```python
from build123d import *

# Parameters (mm, degrees)
SKETCH1_R           = 48.9
SKETCH1_R_2         = 45.9
BOSS_EXTRUDE1_DEPTH = 2
SKETCH2_R           = 1.5
BOSS_EXTRUDE2_DEPTH = 2
SKETCH3_R           = 2.38125
BOSS_EXTRUDE3_DEPTH = 2
FILLET1_R           = 3


with BuildPart() as part:
    # Sketch1 → Boss-Extrude1 (new body)
    with BuildSketch(Plane(origin=(0, 0, 0), x_dir=(1, 0, 0), z_dir=(0, 1, 0))):
        with Locations(Location((0, 0, 0), (0, 0, 270))):
            Circle(SKETCH1_R)
        with Locations(Location((0, 0, 0), (0, 0, 270))):
            Circle(SKETCH1_R_2, mode=Mode.SUBTRACT)
    extrude(amount=BOSS_EXTRUDE1_DEPTH)

    # Sketch2 → Boss-Extrude2 (add)
    # profile 1 of 4: a face of its own
    with BuildSketch(Plane.XZ):
        with BuildLine():
            Line((-3.5, 45.766363194), (-3.5, 42.4))
            ThreePointArc((-3.5, 42.4), (0, 38.9), (3.5, 42.4))
            Line((3.5, 42.4), (3.5, 45.766363194))
            ThreePointArc((3.5, 45.766363194), (0, 45.9), (-3.5, 45.766363194))
        make_face()
        with Locations(Location((0, 42.4, 0), (0, 0, 270))):
            Circle(SKETCH2_R, mode=Mode.SUBTRACT)
    # profile 2 of 4: a face of its own
    with BuildSketch(Plane.XZ):
        with BuildLine():
            ThreePointArc((45.9, 0), (45.866578631, 1.751275164), (45.766363194, 3.5))
            Line((45.766363194, 3.5), (42.4, 3.5))
            ThreePointArc((42.4, 3.5), (38.9, 0), (42.4, -3.5))
            Line((42.4, -3.5), (45.766363194, -3.5))
            ThreePointArc((45.766363194, -3.5), (45.866578631, -1.751275164), (45.9, 0))
        make_face()
        with Locations(Location((42.4, 0, 0), (0, 0, 270))):
            Circle(SKETCH2_R, mode=Mode.SUBTRACT)
    # profile 3 of 4: a face of its own
    with BuildSketch(Plane.XZ):
        with BuildLine():
            Line((-3.5, -42.4), (-3.5, -45.766363194))
            ThreePointArc((-3.5, -45.766363194), (0, -45.9), (3.5, -45.766363194))
            Line((3.5, -45.766363194), (3.5, -42.4))
            ThreePointArc((3.5, -42.4), (0, -38.9), (-3.5, -42.4))
        make_face()
        with Locations(Location((0, -42.4, 0), (0, 0, 270))):
            Circle(SKETCH2_R, mode=Mode.SUBTRACT)
    # profile 4 of 4: a face of its own
    with BuildSketch(Plane.XZ):
        with BuildLine():
            Line((-42.4, 3.5), (-45.766363194, 3.5))
            ThreePointArc((-45.766363194, 3.5), (-45.9, 0), (-45.766363194, -3.5))
            Line((-45.766363194, -3.5), (-42.4, -3.5))
            ThreePointArc((-42.4, -3.5), (-38.9, 0), (-42.4, 3.5))
        make_face()
        with Locations(Location((-42.4, 0, 0), (0, 0, 270))):
            Circle(SKETCH2_R, mode=Mode.SUBTRACT)
    extrude(amount=-BOSS_EXTRUDE2_DEPTH)

    # Sketch3 → Boss-Extrude3 (add)
    with BuildSketch(Plane.XZ):
        with BuildLine():
            ThreePointArc((35.406018707, 29.209995537), (32.456201256, 32.456201256), (29.209995537, 35.406018707))
            Line((29.209995537, 35.406018707), (26.260178086, 32.456201256))
            ThreePointArc((26.260178086, 32.456201256), (26.260178086, 26.260178086), (32.456201256, 26.260178086))
            Line((32.456201256, 26.260178086), (35.406018707, 29.209995537))
        make_face()
        with Locations(Location((29.358189671, 29.358189671, 0), (0, 0, 270))):
            Circle(SKETCH3_R, mode=Mode.SUBTRACT)
    extrude(amount=-BOSS_EXTRUDE3_DEPTH)

    # Fillet1
    fillet1_edges = [part.edges().sort_by_distance(p)[0] for p in [
        (3.5, 1, 45.766363194),
        (-3.5, 1, 45.766363194),
        (45.766363194, 1, -3.5),
        (45.766363194, 1, 3.5),
        (-3.5, 1, -45.766363194),
        (3.5, 1, -45.766363194),
        (-45.766363194, 1, 3.5),
        (-45.766363194, 1, -3.5),
        (35.406018707, 1, 29.209995537),
        (29.209995537, 1, 35.406018707),
    ]]
    fillet(fillet1_edges, radius=FILLET1_R)


solid = part.part
```
Check sheet for the modelled part. Datum: model origin and axes. Units: mm. Give positions to 0.01 mm unless a question says otherwise; leave off trailing zeros. Order: outer loops, then holes, each group sorted by start corner. A loop starts at its lowest first (then second) coordinate and runs counter-clockwise, first axis right, second up. Notation, with made-up numbers: M 20,83.25 L 68,83.25 A18 ccw 68,104.25 Z; hole C 34.5,79.25 d6. An arc over 180 degrees is marked long. Answer in a Markdown table with one row per item. Add a question column.
Q1. Gauge pin test, flat ends, axial feed: pin 1 Ø12 at (x, z) = (16, 33.5) entering from -Y; pin 2 Ø1 at (y, z) = (1, 12) entering from -X. Record the tip position at first contact, or that the pin passes through.
Q2. Thickness scan on L1, parallel to X at y = 1.25, z = 0; L2, parallel to X at y = 1.5, z = 1; L3, parallel to X at y = 0.7, z = 25.5. Record the ranges inside material, lowest first.
Q3. Sectioned sample at D-D, the plane z = -33. Record the boundary of the cut face in (x, y), and give its area (3 significant figures).
Q4. Sectioned sample at A-A, the plane x = 0. Record the boundary of the cut face in (y, z).
Q5. Sectioned sample at B-B, the plane z = 0. Record the boundary of the cut face in (x, y), and give its area (3 significant figures).
Q6. Release check for a two-part mould opening along X. For faces 1 (the cylindrical face through (-4.52, 1.01, 44.66)), 2 (the cylindrical face through (-47.737, 0.986, -10.601)) record: released by +X, released by -X, zero draft, split by the parting line, or undercut.
Q7. Sectioned sample at C-C, the plane x = -18. Record the boundary of the cut face in (y, z), and give its area (3 significant figures).
Verdict:
| question | item | result |
|---|---|---|
| 1 | pin 1 | through |
| 1 | pin 2 | x = -47.53 |
| 2 | L1 | -48.9 to -43.9, -40.9 to -38.9, 38.9 to 40.9, 43.9 to 48.9 |
| 2 | L2 | -48.89 to -43.52, -41.28 to -39.05, 39.05 to 41.28, 43.52 to 48.89 |
| 2 | L3 | -41.72 to -38.16, 27.28 to 31.43, 38.16 to 41.72 |
| 3 | outline | M -36.09,0 L -31.9,0 L -31.9,2 L -36.09,2 Z; M 31.9,0 L 36.09,0 L 36.09,2 L 31.9,2 Z |
| 3 | area | 16.7 mm² |
| 4 | outline | M 0,-48.9 L 2,-48.9 L 2,-43.9 L 0,-43.9 Z; M 0,-40.9 L 2,-40.9 L 2,-38.9 L 0,-38.9 Z; M 0,38.9 L 2,38.9 L 2,40.9 L 0,40.9 Z; M 0,43.9 L 2,43.9 L 2,48.9 L 0,48.9 Z |
| 5 | outline | M -48.9,0 L -43.9,0 L -43.9,2 L -48.9,2 Z; M -40.9,0 L -38.9,0 L -38.9,2 L -40.9,2 Z; M 38.9,0 L 40.9,0 L 40.9,2 L 38.9,2 Z; M 43.9,0 L 48.9,0 L 48.9,2 L 43.9,2 Z |
| 5 | area | 28.0 mm² |
| 6 | face 1 | undercut |
| 6 | face 2 | split by the parting line |
| 7 | outline | M 0,-45.47 L 2,-45.47 L 2,-42.22 L 0,-42.22 Z; M 0,42.22 L 2,42.22 L 2,45.47 L 0,45.47 Z |
| 7 | area | 13.0 mm² |
